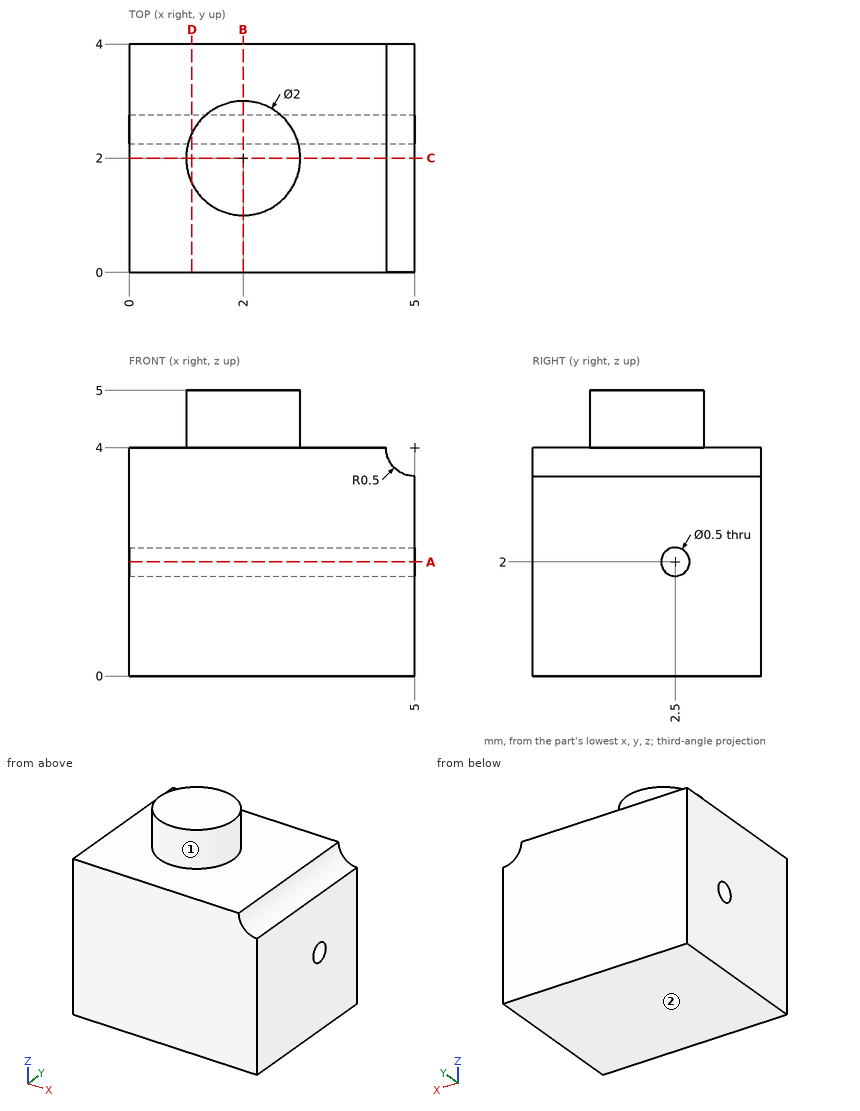
Input: dimensioned drawing with shaded views. Units: mm. Origin: part minimum x, y, z. A direction names the side the tool comes from. Coordinates: 2 decimals unless noted, no trailing zeros. Order: outer loops, then holes, each group sorted by start corner. A loop starts at its lowest first (then second) coordinate and runs counter-clockwise, first axis right, second up. Notation, with made-up numbers: (57.5, 75) - (78.5, 75) arc R12 cw to (78.5, 88) - close; hole circle Ø3 at (74, 42.5). An arc over 180 degrees is marked (long way). One line per item, written item: value.
1) Cut plane B-B on x = 2. Output: boundary loops of the cut face in (y, z).
Computed values:
outline: (0, 0) - (4, 0) - (4, 4) - (3, 4) - (3, 5) - (1, 5) - (1, 4) - (0, 4) - close; hole circle Ø0.5 at (2.5, 2)
2) Cut plane C-C on y = 2. Output: boundary loops of the cut face in (x, z), plus the area to 3 significant figures.
Computed values:
outline: (0, 0) - (5, 0) - (5, 3.5) arc R0.5 cw to (4.5, 4) - (3, 4) - (3, 5) - (1, 5) - (1, 4) - (0, 4) - close
area: 21.8 mm^2
3) Cut plane D-D on x = 1.1. Output: boundary loops of the cut face in (y, z), plus the area to 3 significant figures.
Computed values:
outline: (0, 0) - (4, 0) - (4, 4) - (2.44, 4) - (2.44, 5) - (1.56, 5) - (1.56, 4) - (0, 4) - close; hole circle Ø0.5 at (2.5, 2)
area: 16.7 mm^2
4) Cut plane A-A on z = 2. Output: boundary loops of the cut face in (x, y), plus the area to 3 significant figures.
Computed values:
outline: (0, 0) - (5, 0) - (5, 2.25) - (0, 2.25) - close; (0, 2.75) - (5, 2.75) - (5, 4) - (0, 4) - close
area: 17.5 mm^2
5) Ray query, line 1 (Z direction, x = 1.9, y = 2.5); line 2 (Z direction, x = 3.3, y = 2.5); line 3 (Z direction, x = 4, y = 3.15). Return the intervals inside material, ascending. Write a range as [from, to].
Computed values:
line 1: z = [0, 1.75], [2.25, 5]
line 2: z = [0, 1.75], [2.25, 4]
line 3: z = [0, 4]
6) Reachability of the marked faces 1 and 2 from +Z, -Z, +X, -X, +Y, -Y: full face, straight path, thin tool, end or side. Return the list, or none.
Computed values:
face 1: +Z
face 2: -Z, +X, -X, +Y, -Y
